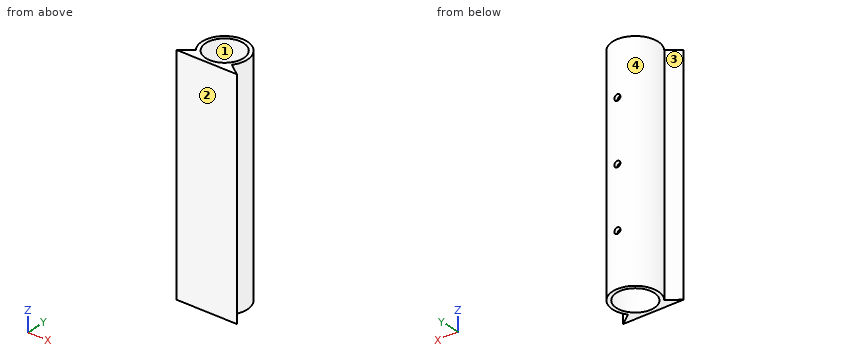
Autodesk Inventor part; units mm, degrees
ref_plane "YZ Plane" through (0, 0, 0) normal (1, 0, 0) x (0, 1, 0)
ref_plane "XZ Plane" through (0, 0, 0) normal (0, 1, 0) x (-1, 0, 0)
ref_plane "XY Plane" through (0, 0, 0) normal (0, 0, 1) x (1, 0, 0)
sketch "Sketch1" plane through (0, 0, 0) normal (0, 1, 0) x (-1, 0, 0)
  line L0 (0, 0) -> (60, 0)
  line L1 (60, 0) -> (60, -150)
  line L2 (60, -150) -> (0, -150)
  line L3 (0, -150) -> (0, 0)
  line L4 (0, 0) -> (40, 0)
  line L5 (40, 0) -> (40, -150)
  line L6 (40, -150) -> (0, -150)
  line L7 (0, -150) -> (0, 0)
  dimension "d0" = 60
  dimension "d1" = 150
  dimension "d2" = 40
extrude "Extrusion1" add sketch "Sketch1" along normal blind 30 contours L0 L5 L2 L3
sketch "Sketch2" plane through (0, 30, 0) normal (0, 1, 0) x (1, 0, 0)
  line L0 (0, 150) -> (-40, 150)
  line L1 (-20, 150) -> (-20, 0)
  line L2 (-20, 0) -> (-20, 75)
  line L3 (-20, 75) -> (-20, 150)
  line L4 (-20, 75) -> (-20, 115)
  line L5 (-20, 75) -> (-20, 35)
  line L6 (-20, 35) -> (-20, 115)
  circle A0 centre (-20, 35) radius 1.65
  circle A1 centre (-20, 75) radius 1.75
  circle A2 centre (-20, 35) radius 1.75
  circle A3 centre (-20, 115) radius 1.75
  circle A4 centre (-20, 35) radius 2
  circle A5 centre (-20, 75) radius 2
  circle A6 centre (-20, 115) radius 2
  point P0 (0, 0)
  dimension "d5" = 40
  dimension "d6" = 40
  dimension "d7" = 3.3
  dimension "d8" = 3.5
  dimension "d9" = 3.5
  dimension "d10" = 3.5
  dimension "d11" = 4
  dimension "d12" = 4
  dimension "d13" = 4
extrude "Extrusion2" cut sketch "Sketch2" against normal blind 4
sketch "Sketch3" plane through (-40, 0, 0) normal (0, 0, 1) x (1, 0, 0)
  line L0 (0, 0) -> (0, 30)
  line L1 (40, 0) -> (40, 30)
  line L2 (0, 30) -> (40, 30)
  line L3 (40, 30) -> (40, 15)
  line L4 (40, 15) -> (0, 15)
  line L5 (0, 15) -> (0, 30)
  line L6 (0, 0) -> (40, 0)
  line L7 (40, 15) -> (20, 15)
  line L8 (20, 15) -> (20, 0)
  line L9 (20, 0) -> (40, 0)
  line L10 (40, 0) -> (40, 15)
  circle A0 centre (20, 15) radius 15
  line L11 (0, 0) -> (40, 0)
  line L12 (40, 0) -> (40, -5)
  line L13 (40, -5) -> (0, -5)
  line L14 (0, -5) -> (0, 0)
  circle A1 centre (20, 15) radius 12.5
  line L15 (20, 15) -> (0, 0)
  line L16 (20, 15) -> (40, 0)
  point P0 (20, 30)
  point P1 (32, 6)
  point P2 (8, 6)
  dimension "d16" = 30
  dimension "d17" = 5
  dimension "d18" = 25
extrude "Extrusion3" cut sketch "Sketch3" against normal blind 150 contours L0 L4 A0 L15 | L0 L2 A0 L4 | L16 A0 L4 L1 | A1 L15 L8 | L8 L16 A1 | A1 L4 L15 | L2 L1 L4 A0 | A1 L4 | L4 A1 L16
properties part number "Pin Cylinder"
Input: part model. Units: mm. Frame: model coordinates. Face numbers are marked on the shaded views. A direction names the side the tool comes from. Coordinates: 2 decimals unless noted, no trailing zeros. Order: outer loops, then holes, each group sorted by start corner. A loop starts at its lowest first (then second) coordinate and runs counter-clockwise, first axis right, second up. Notation, with made-up numbers: M 4,20.25 L 29,20.25 A14 ccw 29,34.25 Z; hole C 78.5,15.25 d11. An arc over 180 degrees is marked long. Answer in a Markdown table with one row per item.
(1) Section query A-A, the plane y = 15. Output: boundary loops of the cut face in (x, z), plus the area to 3 significant figures.
Numbers:
| item | result |
|---|---|
| outline | M -35,-150 L -32.5,-150 L -32.5,0 L -35,0 Z; M -7.5,-150 L -5,-150 L -5,0 L -7.5,0 Z |
| area | 750 mm^2 |
(2) Draft query along Y for the marked faces 1 and 2. Return one class per face: pulls with the +Y half, pulls with the -Y half, needs draft (parallel to the pull), parting line crosses it, or undercut.
Numbers:
| item | result |
|---|---|
| face 1 | undercut |
| face 2 | pulls with the -Y half |
(3) Access query for the marked faces 3 and 4. Directions: +Z, -Z, +X, -X, +Y, -Y. A direction counts if a zero-diameter tool reaches every point of the face in a straight line with its end or side. Return the directions, or none.
Numbers:
| item | result |
|---|---|
| face 3 | +Z, -Z, -X |
| face 4 | +Z, -Z |
(4) Contact query for flat-ended pins moving along their axis: pin 1 Ø5 at (x, z) = (-20, -115) entering from +Y; pin 2 Ø4 at (y, z) = (17, -103) entering from -X; pin 3 Ø3 at (y, z) = (12, -103.5) entering from -X; pin 4 Ø10 at (y, z) = (22.5, -111) entering from -X. Output: stop coordinate, or through.
Numbers:
| item | result |
|---|---|
| pin 1 | stops at y = 30 |
| pin 2 | stops at x = -35 |
| pin 3 | stops at x = -34.92 |
| pin 4 | stops at x = -34.79 |
(5) Section query D-D, the plane x = -12. Output: boundary loops of the cut face in (y, z).
Numbers:
| item | result |
|---|---|
| outline | M 0,-150 L 5.4,-150 L 5.4,0 L 0,0 Z; M 24.6,-150 L 27.69,-150 L 27.69,0 L 24.6,0 Z |
(6) Section query B-B, the plane x = -20. Output: boundary loops of the cut face in (y, z).
Numbers:
| item | result |
|---|---|
| outline | M 0,-150 L 2.5,-150 L 2.5,0 L 0,0 Z; M 27.5,-150 L 30,-150 L 30,-117 L 27.5,-117 Z; M 27.5,-113 L 30,-113 L 30,-77 L 27.5,-77 Z; M 27.5,-73 L 30,-73 L 30,-37 L 27.5,-37 Z; M 27.5,-33 L 30,-33 L 30,0 L 27.5,0 Z |
(7) Section query C-C, the plane z = -28. Output: boundary loops of the cut face in (x, y).
Numbers:
| item | result |
|---|---|
| outline | M -40,0 L 0,0 L -8,6 A15 ccw long -32,6 Z; hole C -20,15 d25 |
(8) Material intervals for line 1 (Z direction, x = -20, y = 28); line 2 (X direction, y = 15, z = -54); line 3 (Y direction, x = -6.5, z = -35) (3 decimals), sorted ascending. Write a range as [from, to].
Numbers:
| item | result |
|---|---|
| line 1 | z = [-150, -117], [-113, -77], [-73, -37], [-33, 0] |
| line 2 | x = [-35, -32.5], [-7.5, -5] |
| line 3 | y = [0, 4.875], [8.462, 21.538] |
